Part model, mm, in its own coordinate system. Face numbers are marked on the shaded views. A direction names the side the tool comes from. Round coordinates to 2 decimals unless told otherwise and drop trailing zeros. Order: outer loops, then holes, each group sorted by start corner. A loop starts at its lowest first (then second) coordinate and runs counter-clockwise, first axis right, second up. Notation, with made-up numbers: (26.5, -22.75) - (78.5, -22.75) arc R17 cw to (78.5, 4.25) - close; hole circle Ø2 at (-13.75, -5.5). An arc over 180 degrees is marked (long way). Answer as a JSON object with one key per item and string values.
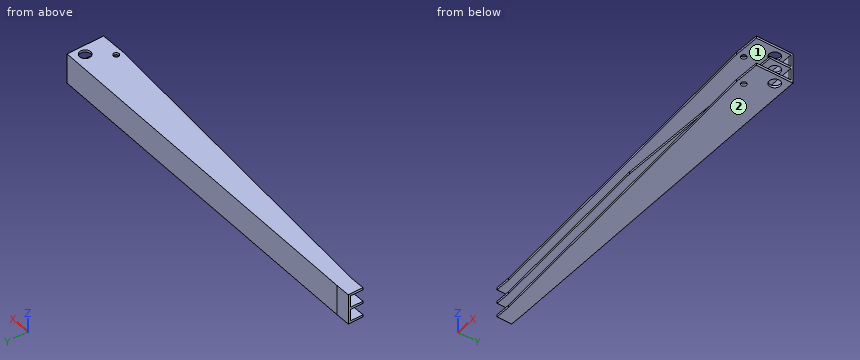
```python
from build123d import *

# Parameters (mm, degrees)
BOSS_EXTRUDE1_DEPTH      = 15
BOSS_EXTRUDE2_DEPTH      = 15
BOSS_EXTRUDE3_DEPTH      = 192.8
BOSS_EXTRUDE4_DEPTH      = 7.5
BOSS_EXTRUDE4_DEPTH_BACK = 7.5
SKETCH5_R                = 38.1
SKETCH5_R_2              = 19.05
CUT_EXTRUDE1_DEPTH       = 2627.039580814
CUT_EXTRUDE2_DEPTH       = 15


with BuildPart() as part:
    # Sketch1 → Boss-Extrude1 (new body)
    with BuildSketch(Plane.XY):
        Polygon((-2600, 304.8), (-2498.4, 304.8), (0, 254), (0, 0), (-177.8, 0), (-2498.4, 203.2), (-2600, 203.2), align=None)
    extrude(amount=-BOSS_EXTRUDE1_DEPTH)



with BuildPart() as body_2:
    # Sketch2 → Boss-Extrude2 (new body)
    with BuildSketch(Plane.XY.offset(177.8)):
        Polygon((-2498.4, 203.2), (-177.8, 0), (0, 0), (0, 254), (-2498.4, 304.8), (-2600, 304.8), (-2600, 203.2), align=None)
    extrude(amount=BOSS_EXTRUDE2_DEPTH)


with BuildPart() as part_1:
    add(part.part)

    add(body_2.part)  # Boss-Extrude3 merges body 2
    # Sketch3 → Boss-Extrude3 (add)
    with BuildSketch(Plane.XY.offset(192.8)):
        Polygon((-2600, 289.8), (-2600, 304.8), (-2498.4, 304.8), (0, 254), (0, 238.996899585), (-15, 239.301894782), (-2498.55248184, 289.8), align=None)
    extrude(amount=-BOSS_EXTRUDE3_DEPTH)

    # Sketch6 → Boss-Extrude4 (add, two sides: drawn at the far end of the back side and taken through both)
    with BuildSketch(Plane.XY.offset(88.9).offset(-BOSS_EXTRUDE4_DEPTH_BACK)):
        Polygon((-2498.4, 203.2), (-177.8, 0), (0, 0), (0, 254), (-2498.4, 304.8), (-2600, 304.8), (-2600, 203.2), align=None)
    extrude(amount=BOSS_EXTRUDE4_DEPTH + BOSS_EXTRUDE4_DEPTH_BACK)

    # Sketch5 → Cut-Extrude1 (cut, through all)
    with BuildSketch(Plane.XY.offset(192.8)):
        with Locations((-63.5, 176.782795882)):
            Circle(SKETCH5_R)
        with Locations((-171.45, 44.45)):
            Circle(SKETCH5_R_2)
    extrude(amount=-CUT_EXTRUDE1_DEPTH, mode=Mode.SUBTRACT)

    # Sketch7 → Cut-Extrude2 (cut)
    with BuildSketch(Plane.XY.offset(96.4)):
        Polygon((-1265.58125, 95.25), (0, 95.25), (0, 0), (-177.8, 0), align=None)
    extrude(amount=-CUT_EXTRUDE2_DEPTH, mode=Mode.SUBTRACT)


solid = part_1.part
```
Item 1: Cut at D-D (x = -1339.5). Write the cut outline in (y, z), plus the area to 3 significant figures.
Taken from the geometry:
{"outline": "(101.72, -15) - (281.24, -15) - (281.24, 192.8) - (101.72, 192.8) - (101.72, 177.8) - (266.23, 177.8) - (266.23, 96.4) - (101.72, 96.4) - (101.72, 81.4) - (266.23, 81.4) - (266.23, 0) - (101.72, 0) - close", "area": "10,500 mm2"}
Item 2: Cut at C-C (x = -653). Write the cut outline in (y, z).
Taken from the geometry:
{"outline": "(41.61, -15) - (267.28, -15) - (267.28, 192.8) - (41.61, 192.8) - (41.61, 177.8) - (252.27, 177.8) - (252.27, 96.4) - (95.25, 96.4) - (95.25, 81.4) - (252.27, 81.4) - (252.27, 0) - (41.61, 0) - close"}
Item 3: Probe L1, parallel to Z at x = -653.5, y = 99.5; L2, parallel to Z at x = -709, y = 70; L3, parallel to Y at x = -63.5, z = -8. List the from-to ranges inside material, lowest first. Write a range as from..to.
Taken from the geometry:
{"L1": "-15..0, 81.4..96.4, 177.8..192.8", "L2": "-15..0, 177.8..192.8", "L3": "0..138.68, 214.88..255.29"}
Item 4: Tool access for the marked faces 1 and 2: list every direction of +Z, -Z, +X, -X, +Y, -Y with a clear straight run to the whole face (end or side of a thin tool).
Taken from the geometry:
{"face 1": "-X, -Y", "face 2": "-Z, +X, -X, +Y, -Y"}
Item 5: Cut at B-B (z = 37). Write the cut outline in (x, y), plus the area to 3 significant figures.
Taken from the geometry:
{"outline": "(-2600, 289.8) - (-2498.55, 289.8) - (0, 239) - (0, 254) - (-2498.4, 304.8) - (-2600, 304.8) - close", "area": "39,000 mm2"}
Item 6: Drop flat-ended pins along their axis: P1, Ø4.5, axis at x = -2528, z = 183, coming from the -Y side; P2, Ø8, axis at x = -873.5, z = 80, coming from the +Y side; P3, Ø12, axis at x = -893.5, z = 90, coming from the -Y side. Give the stop position or say it passes through.
Taken from the geometry:
{"P1": "y = 203.2", "P2": "y = 271.84", "P3": "y = 95.25"}
Item 7: Cut at A-A (x = -63.5). Write the cut outline in (y, z), plus the area to 3 significant figures.
Taken from the geometry:
{"outline": "(0, -15) - (138.68, -15) - (138.68, 0) - (0, 0) - close; (0, 177.8) - (138.68, 177.8) - (138.68, 192.8) - (0, 192.8) - close; (95.25, 81.4) - (138.68, 81.4) - (138.68, 96.4) - (95.25, 96.4) - close; (214.88, -15) - (255.29, -15) - (255.29, 192.8) - (214.88, 192.8) - (214.88, 177.8) - (240.29, 177.8) - (240.29, 96.4) - (214.88, 96.4) - (214.88, 81.4) - (240.29, 81.4) - (240.29, 0) - (214.88, 0) - close", "area": "9,070 mm2"}
